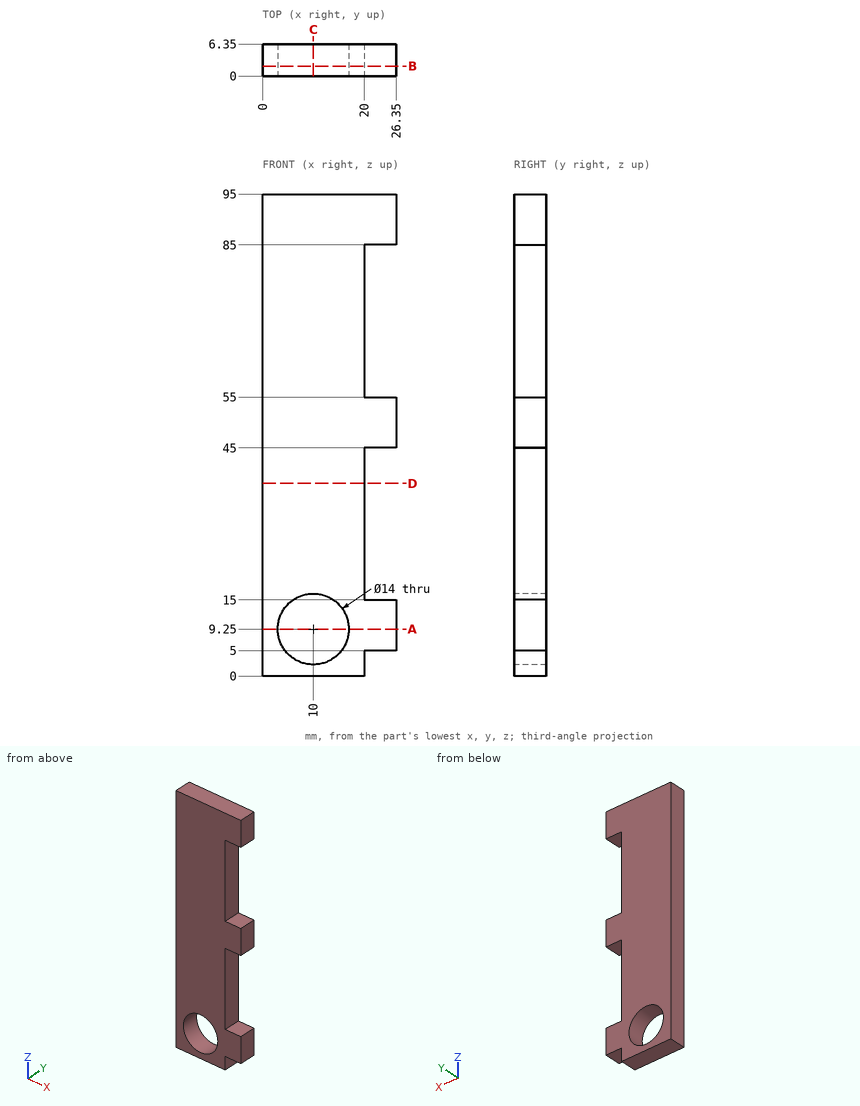
Print and shaded views of the part. All mm, measured from the part's lowest x, y and z. Coordinates: 2 decimals unless noted, no trailing zeros. Order: outer loops, then holes, each group sorted by start corner. A loop starts at its lowest first (then second) coordinate and runs counter-clockwise, first axis right, second up.
(1) Slice it at B-B, the plane y = 2. Write the cut outline in (x, z), and give its area (3 significant figures).
Check sheet entries:
outline: (0, 0) - (20, 0) - (20, 5) - (26.35, 5) - (26.35, 15) - (20, 15) - (20, 45) - (26.35, 45) - (26.35, 55) - (20, 55) - (20, 85) - (26.35, 85) - (26.35, 95) - (0, 95) - close; hole circle Ø14 at (10, 9.25)
area: 1,940 mm2
(2) Pin check, flat tip, straight feed: pin 1 Ø1.9 at (x, y) = (24.5, 2.5) entering from -Z. Stop position of the tip, or through.
Check sheet entries:
pin 1: stops at z = 5
(3) Slice it at C-C, the plane x = 10. Write the cut outline in (y, z).
Check sheet entries:
outline: (0, 0) - (6.35, 0) - (6.35, 2.25) - (0, 2.25) - close; (0, 16.25) - (6.35, 16.25) - (6.35, 95) - (0, 95) - close
(4) Probe L1, parallel to Z at x = 23, y = 3.75; L2, parallel to X at y = 2.25, z = 9.25; L3, parallel to X at y = 2.25, z = 68. List the from-to ranges inside material, lowest first.
Check sheet entries:
L1: z = 5 to 15, 45 to 55, 85 to 95
L2: x = 0 to 3, 17 to 26.35
L3: x = 0 to 20
(5) Slice it at D-D, the plane z = 38. Write the cut outline in (x, y), and give its area (3 significant figures).
Check sheet entries:
outline: (0, 0) - (20, 0) - (20, 6.35) - (0, 6.35) - close
area: 127 mm2
(6) Slice it at A-A, the plane z = 9.25. Write the cut outline in (x, y), and give its area (3 significant figures).
Check sheet entries:
outline: (0, 0) - (3, 0) - (3, 6.35) - (0, 6.35) - close; (17, 0) - (26.35, 0) - (26.35, 6.35) - (17, 6.35) - close
area: 78.4 mm2
